Source: CAD feature listing. Evaluate the final solid. Frame: model axes, mm. A direction names the side the tool comes from. Round coordinates to 2 decimals unless told otherwise and drop trailing zeros. Loops run counter-clockwise (first coordinate to the right, second up) from the corner with the lowest first, then second, coordinate; pieces in that order, holes last. Notation, with made-up numbers: (60, -4.5) - (64, -4.5) arc R18 cw to (64, 21.5) - close; hole circle Ø9 at (22.5, 46.5). An arc over 180 degrees is marked (long way). One line per question, with ' | ' between items.
from build123d import *

# Parameters (mm, degrees)
SKETCH3_R           = 2.025729463
BOSS_EXTRUDE1_DEPTH = 74.168
BOSS_EXTRUDE5_START = -16.51
SKETCH4_R           = 9.333271044
BOSS_EXTRUDE5_DEPTH = 12.7


with BuildPart() as part:
    # Sketch1 → Revolve1 (revolve)
    with BuildSketch(Plane(origin=(0, 0, 0), x_dir=(1, 0, 0), z_dir=(0, 1, 0))):
        with BuildLine():
            Line((-16.919904062, 26.957438718), (-5.784386472, 15.821921128))
            ThreePointArc((-5.784386472, 15.821921128), (-5.784386472, 26.957438718), (-16.919904062, 26.957438718))
        make_face()
    revolve(axis=Axis((-16.919904062, 0, -26.957438718), (0.7071067811865476, 0, 0.7071067811865476)))

    # Sketch3 → Boss-Extrude1 (add)
    with BuildSketch(Plane(origin=(0, 0, 0), x_dir=(1, 0, 0), z_dir=(0, 1, 0))):
        with Locations(Location((-11.072249639, 21.554324411, 0), (0, 0, 134.105346527))):
            Circle(SKETCH3_R)
    extrude(amount=BOSS_EXTRUDE1_DEPTH)

    # Sketch4 → Boss-Extrude5 (add)
    with BuildSketch(Plane(origin=(0, 0, 0), x_dir=(0, 0, -1), z_dir=(1, 0, 0)).offset(BOSS_EXTRUDE5_START)):
        with Locations((21.554324411, 76.835)):
            Circle(SKETCH4_R)
        Polygon((22.443324411, 75.946), (22.443324411, 74.168), (20.665324411, 74.168), (20.665324411, 75.946), (18.887324411, 75.946), (18.887324411, 77.724), (20.665324411, 77.724), (20.665324411, 79.502), (22.443324411, 79.502), (22.443324411, 77.724), (24.221324411, 77.724), (24.221324411, 75.946), align=None, mode=Mode.SUBTRACT)
    extrude(amount=BOSS_EXTRUDE5_DEPTH)


solid = part.part
1. Section query A-A, the plane x = -14.75. Return loops of the section in (y, z) (3 decimals), plus the area to 3 significant figures.
Worked out:
outline: circle Ø14.206 at (0, -21.39); circle Ø18.667 at (76.835, -21.554); hole (74.168, -22.443) - (75.946, -22.443) - (75.946, -24.221) - (77.724, -24.221) - (77.724, -22.443) - (79.502, -22.443) - (79.502, -20.665) - (77.724, -20.665) - (77.724, -18.887) - (75.946, -18.887) - (75.946, -20.665) - (74.168, -20.665) - close | area: 416 mm2
2. Section query B-B, the plane z = -25.5. Return loops of the section in (x, y), plus the area to 3 significant figures.
Worked out:
outline: circle Ø13.43 at (-11.35, 0); (-16.51, 68.38) - (-3.81, 68.38) - (-3.81, 85.29) - (-16.51, 85.29) - close | area: 357 mm2
3. Material intervals for probe 1 along Y at (x, z) = (-15.5, -24); probe 2 along Z at (x, y) = (-15.75, 75); probe 3 along Z at (x, y) = (-5.5, 79), sorted ascending.
Worked out:
probe 1: y = -6.16 to 6.16, 67.83 to 75.95, 77.72 to 85.84 | probe 2: z = -30.71 to -22.44, -20.67 to -12.4 | probe 3: z = -30.63 to -22.44, -20.67 to -12.48
4. Section query C-C, the plane x = -11.25. Return loops of the section in (y, z) (3 decimals), plus the area to 3 significant figures.
Worked out:
outline: (7.565, -23.572) - (67.722, -23.572) arc R9.333 ccw (long way) to (67.722, -19.536) - (7.652, -19.536) arc R7.873 ccw (long way) to start; hole (74.168, -22.443) - (75.946, -22.443) - (75.946, -24.221) - (77.724, -24.221) - (77.724, -22.443) - (79.502, -22.443) - (79.502, -20.665) - (77.724, -20.665) - (77.724, -18.887) - (75.946, -18.887) - (75.946, -20.665) - (74.168, -20.665) - close | area: 694 mm2
5. Section query D-D, the plane y = 36. Return loops of the section in (x, z).
Worked out:
outline: circle Ø4.05 at (-11.07, -21.55)
6. Contact query for flat-ended pins moving along their axis: P1, Ø2, axis at x = -13, y = 75.5, coming from the +Z side; P2, Ø3, axis at y = 53, z = -24, coming from the -X side; P3, Ø0.9, axis at x = -13.5, z = -20, coming from the +Y side. Output: stop coordinate, or through.
Worked out:
P1: stops at z = -12.23 | P2: stops at x = -12.86 | P3: stops at y = 86.1
7. Mould query, pull axis Y, two halves, no side actions, for faces 4 (the flat face through (-10, 77.724, -20)), 5 (the flat face through (-3.81, 75, -23)). Classes: released by +Y, released by -Y, zero draft, split by the parting line, or undercut.
Worked out:
face 4: undercut | face 5: zero draft
8. Access query for faces 1 (the flat face through (-16.51, 75, -23)), 2 (the cylindrical face through (-10.432, 37.198, -23.476)), 3 (the flat face through (-10, 77, -18.887)). Directions: +Z, -Z, +X, -X, +Y, -Y. A direction counts if a zero-diameter tool reaches every point of the face in a straight line with its end or side. Return the directions, or none.
Worked out:
face 1: +Z, -Z, -X, +Y | face 2: none | face 3: +X, -X
